Design review of the part shown in the three views and the two pictorial views. Dimensions are in mm from the part's minimum x, y and z. Round coordinates to 2 decimals unless told otherwise and drop trailing zeros. Order: outer loops, then holes, each group sorted by start corner. A loop starts at its lowest first (then second) coordinate and runs counter-clockwise, first axis right, second up.
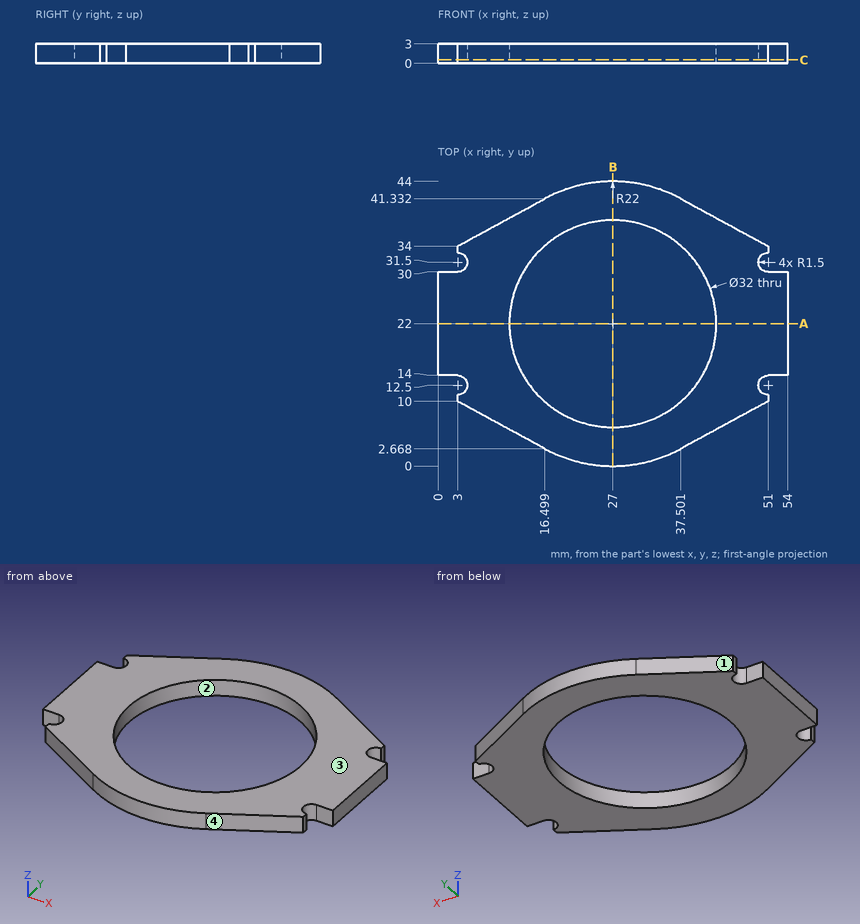
(1) Consider section C-C (z = 0.55). Write out the cut boundary in (x, y).
Data:
outline: (0, 14) - (3, 14) arc R1.5 cw to (3, 11) - (3, 10) - (16.5, 2.67) arc R22 ccw to (37.5, 2.67) - (51, 10) - (51, 11) arc R1.5 cw to (51, 14) - (54, 14) - (54, 30) - (51, 30) arc R1.5 cw to (51, 33) - (51, 34) - (37.5, 41.33) arc R22 ccw to (16.5, 41.33) - (3, 34) - (3, 33) arc R1.5 cw to (3, 30) - (0, 30) - close; hole circle Ø32 at (27, 22)
(2) Draft analysis for pull direction X (two halves, no side actions). For the marked faces 1, 2, 3 and 4, state which applies: pulls with the +X half, pulls with the -X half, needs draft (parallel to the pull), parting line crosses it, or undercut.
Data:
face 1: pulls with the -X half
face 2: undercut
face 3: needs draft
face 4: pulls with the +X half
(3) To check wall thickness, follow probe 1 along Y at (x, z) = (27, 1.35); probe 2 along X at (y, z) = (11.5, 0.6) (1 decimal); probe 3 along Y at (x, z) = (37, 1.85) (1 decimal). State the ranges of each line that lie inside material, in increasing order.
Data:
probe 1: y = 0 to 6, 38 to 44
probe 2: x = 4.1 to 14.9, 39.1 to 49.9
probe 3: y = 2.4 to 9.5, 34.5 to 41.6
(4) Insertion check: pin 1 (0.9 mm diameter, centred on x = 52.5, z = 1.5, fed in from +Y); pin 2 (0.8 mm diameter, centred on y = 33.5, z = 2, fed in from +X); pin 3 (0.9 mm diameter, centred on x = 1, z = 2, fed in from -Y); pin 4 (5 mm diameter, centred on x = 34, y = 10.5, fed in from +Z). Each pin has a flat end and moves straight along its axis. Give the tip position at first contact, or say it passes through.
Data:
pin 1: stops at y = 30
pin 2: stops at x = 51
pin 3: stops at y = 14
pin 4: passes through
(5) Consider section A-A (y = 22). Write out the cut boundary in (x, z).
Data:
outline: (0, 0) - (11, 0) - (11, 3) - (0, 3) - close; (43, 0) - (54, 0) - (54, 3) - (43, 3) - close
(6) Consider section B-B (x = 27). Write out the cut boundary in (y, z).
Data:
outline: (0, 0) - (6, 0) - (6, 3) - (0, 3) - close; (38, 0) - (44, 0) - (44, 3) - (38, 3) - close
